from build123d import *

# Parameters (mm, degrees)
ESQUISSE1_W             = 40
ESQUISSE1_H             = 3
BOSS_EXTRU_1_DEPTH      = 338
ESQUISSE2_W             = 7.35
ESQUISSE2_H             = 6
ESQUISSE2_W_2           = 9.3
ENL_V_MAT_EXTRU_1_DEPTH = 6
ESQUISSE3_W             = 6
ESQUISSE3_H             = 3
BOSS_EXTRU_2_DEPTH      = 6
ESQUISSE4_W             = 6
ESQUISSE4_H             = 6
ENL_V_MAT_EXTRU_2_DEPTH = 6


with BuildPart() as part:
    # Esquisse1 → Boss.-Extru.1 (new body)
    with BuildSketch(Plane.XY):
        with Locations((20, 1.5)):
            Rectangle(ESQUISSE1_W, ESQUISSE1_H)
    extrude(amount=BOSS_EXTRU_1_DEPTH)

    # Esquisse2 → Enlèv. mat.-Extru.1 (cut)
    with BuildSketch(Plane(origin=(0, 3, 0), x_dir=(1, 0, 0), z_dir=(0, 1, 0))):
        with Locations((3.675, -295)):
            Rectangle(ESQUISSE2_W, ESQUISSE2_H)
        with Locations((20, -295)):
            Rectangle(ESQUISSE2_W_2, ESQUISSE2_H)
        with Locations((36.325, -295)):
            Rectangle(ESQUISSE2_W, ESQUISSE2_H)
    extrude(amount=-ENL_V_MAT_EXTRU_1_DEPTH, mode=Mode.SUBTRACT)

    # Esquisse3 → Boss.-Extru.2 (add)
    with BuildSketch(Plane.XY.offset(338)):
        with Locations((3, 1.5)):
            Rectangle(ESQUISSE3_W, ESQUISSE3_H)
        with Locations((20, 1.5)):
            Rectangle(ESQUISSE3_W, ESQUISSE3_H)
        with Locations((37, 1.5)):
            Rectangle(ESQUISSE3_W, ESQUISSE3_H)
    boss_extru_2 = extrude(amount=BOSS_EXTRU_2_DEPTH)

    # Symétrie1: Boss.-Extru.2 across plane
    add(boss_extru_2.mirror(Plane.XY.offset(169)))

    # Esquisse4 → Enlèv. mat.-Extru.2 (cut)
    with BuildSketch(Plane.XZ):
        with Locations((3, 341)):
            Rectangle(ESQUISSE4_W, ESQUISSE4_H)
    extrude(amount=-ENL_V_MAT_EXTRU_2_DEPTH, mode=Mode.SUBTRACT)


solid = part.part
Could you check a few things on this model? Use its own coordinates, in mm. Round coordinates to 2 decimals unless told otherwise and drop trailing zeros. Write each loop counter-clockwise with the first axis right and the second up, starting at its lowest first coordinate (ties: lowest second). Pieces come first, ordered by that corner, then holes. Notation, with made-up numbers: (-22, 41.5) -> (-3, 41.5) arc R25 ccw to (-3, 73.5) -> close; hole circle Ø10 at (-2, 22.25). An arc over 180 degrees is marked (long way). Use a Markdown table: item, result.
1. If we section it at B-B (x = 10.5): List the corners of the cut face in (y, z) for me.
Answer key:
| item | result |
|---|---|
| outline | (0, 0) -> (3, 0) -> (3, 338) -> (0, 338) -> close |
2. For pin 1 Ø1.5 at (x, y) = (10, 1.5) entering from -Z; pin 2 Ø1.5 at (y, z) = (2, 341) entering from -X; pin 3 Ø1.5 at (y, z) = (1.5, 295.5) entering from -X, each with a flat end and sliding along its axis, tell me the tip position at first contact or that it passes through.
Answer key:
| item | result |
|---|---|
| pin 1 | stops at z = 0 |
| pin 2 | stops at x = 17 |
| pin 3 | stops at x = 7.35 |
3. Please list where these lines run through material, in increasing order: probe 1 along Z at (x, y) = (38, 0.35); probe 2 along Z at (x, y) = (15.5, 0.3); probe 3 along Z at (x, y) = (31.5, 2.7).
Answer key:
| item | result |
|---|---|
| probe 1 | z = -6 to 292, 298 to 344 |
| probe 2 | z = 0 to 292, 298 to 338 |
| probe 3 | z = 0 to 338 |
